```python
from build123d import *

# Parameters (mm, degrees)
SKETCH1_R             = 1.6
BOSS_EXTRUDE2_DEPTH   = 25
BOSS_EXTRUDE2_2_DEPTH = 25
BOSS_EXTRUDE2_3_DEPTH = 25
BOSS_EXTRUDE2_4_DEPTH = 25
BOSS_EXTRUDE4_DEPTH   = 5


with BuildPart() as part:
    # Sketch1 → Boss-Extrude2 (new body)
    with BuildSketch(Plane.XY):
        with Locations((-28.14771299, -24.13)):
            Circle(SKETCH1_R)
    extrude(amount=BOSS_EXTRUDE2_DEPTH)



with BuildPart() as body_2:
    # Sketch1 → Boss-Extrude2 2 (new body)
    with BuildSketch(Plane.XY):
        with Locations((40.977777778, -8.89)):
            Circle(SKETCH1_R)
    extrude(amount=BOSS_EXTRUDE2_2_DEPTH)


with BuildPart() as body_3:
    # Sketch1 → Boss-Extrude2 3 (new body)
    with BuildSketch(Plane.XY):
        with Locations((40.977777778, 19.05)):
            Circle(SKETCH1_R)
    extrude(amount=BOSS_EXTRUDE2_3_DEPTH)


with BuildPart() as body_4:
    # Sketch1 → Boss-Extrude2 4 (new body)
    with BuildSketch(Plane.XY):
        with Locations(Location((-28.14771299, 24.13, 0), (0, 0, 180))):
            Circle(SKETCH1_R)
    extrude(amount=BOSS_EXTRUDE2_4_DEPTH)


with BuildPart() as part_1:
    add(part.part)

    add(body_2.part)  # Boss-Extrude4 merges body 2

    add(body_3.part)  # Boss-Extrude4 merges body 3

    add(body_4.part)  # Boss-Extrude4 merges body 4
    # Sketch1_6 → Boss-Extrude4 (add)
    with BuildSketch(Plane.XY):
        with BuildLine():
            Line((-24.266666667, 25.67), (-24.266666667, 22.066666667))
            ThreePointArc((-24.266666667, 22.066666667), (-23.973773448, 21.359559885), (-23.266666667, 21.066666667))
            Line((-23.266666667, 21.066666667), (42.38771299, 21.066666667))
            ThreePointArc((42.38771299, 21.066666667), (43.094819771, 20.773773448), (43.38771299, 20.066666667))
            Line((43.38771299, 20.066666667), (43.38771299, -15.318617799))
            ThreePointArc((43.38771299, -15.318617799), (43.094819771, -16.02572458), (42.38771299, -16.318617799))
            Line((42.38771299, -16.318617799), (-25.54771299, -16.318617799))
            ThreePointArc((-25.54771299, -16.318617799), (-26.254819771, -16.611511017), (-26.54771299, -17.318617799))
            Line((-26.54771299, -17.318617799), (-26.54771299, -24.13))
            Line((-26.54771299, -24.13), (-26.54771299, -25.67))
            ThreePointArc((-26.54771299, -25.67), (-26.840606209, -26.377106781), (-27.54771299, -26.67))
            Line((-27.54771299, -26.67), (-38.38771299, -26.67))
            ThreePointArc((-38.38771299, -26.67), (-41.923246896, -25.205533906), (-43.38771299, -21.67))
            Line((-43.38771299, -21.67), (-43.38771299, 21.67))
            ThreePointArc((-43.38771299, 21.67), (-41.923246896, 25.205533906), (-38.38771299, 26.67))
            Line((-38.38771299, 26.67), (-25.266666667, 26.67))
            ThreePointArc((-25.266666667, 26.67), (-24.559559885, 26.377106781), (-24.266666667, 25.67))
        make_face()
    extrude(amount=-BOSS_EXTRUDE4_DEPTH)


solid = part_1.part
```
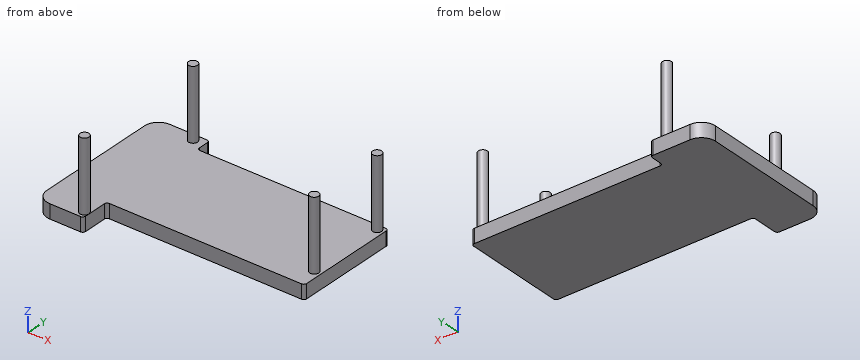
Build history of the part. All positions in model axes, mm. Give positions to 0.01 mm unless a question says otherwise; leave off trailing zeros. Loops run counter-clockwise (first coordinate to the right, second up) from the corner with the lowest first, then second, coordinate; pieces in that order, holes last.
Item 1: Slice it at D-D, the plane y = 9.5. List the corners of the cut face in (x, z), and give its area (3 significant figures).
Answers follow:
outline: (-43.39, -5) - (43.39, -5) - (43.39, 0) - (-43.39, 0) - close
area: 434 mm2
Item 2: Flat gauge pins, fed straight in: pin 1 (8 mm diameter, centred on y = -21, z = 19, fed in from -X); pin 2 (2.5 mm diameter, centred on x = 15.5, z = -2.5, fed in from +Y); pin 3 (5 mm diameter, centred on x = -1.5, y = 19.5, fed in from +Z). Where does each tip first touch, or does it go through?
Answers follow:
pin 1: stops at x = -29.75
pin 2: stops at y = 21.07
pin 3: stops at z = 0
Item 3: Slice it at A-A, the plane y = 19.05. List the corners of the cut face in (x, z).
Answers follow:
outline: (-43.39, -5) - (43.39, -5) - (43.39, 0) - (42.58, 0) - (42.58, 25) - (39.38, 25) - (39.38, 0) - (-43.39, 0) - close
Item 4: Slice it at C-C, the plane x = -3.5. List the corners of the cut face in (y, z).
Answers follow:
outline: (-16.32, -5) - (21.07, -5) - (21.07, 0) - (-16.32, 0) - close
Item 5: Drill centre lines: line 1 (Z direction, x = 10, y = 4.5); line 2 (X direction, y = -9, z = 11.25); line 3 (Y direction, x = 24, z = -0.75). Where is each one in solid material? Low to high.
Answers follow:
line 1: z = -5 to 0
line 2: x = 39.38 to 42.57
line 3: y = -16.32 to 21.07
Item 6: Slice it at B-B, the plane z = 1.5. List the corners of the cut face in (x, y), and give its area (3 significant figures).
Answers follow:
outline: circle Ø3.2 at (-28.15, -24.13); circle Ø3.2 at (-28.15, 24.13); circle Ø3.2 at (40.98, -8.89); circle Ø3.2 at (40.98, 19.05)
area: 32.2 mm2
